```python
from build123d import *

# Parameters (mm, degrees)
OUTLINE_DEPTH        = 1.6
FILLETS_R            = 0.8
FILLET2_R            = 2
SKETCH3_R            = 8.5
LED_RING_AREA_DEPTH  = 1
SKETCH4_R            = 1.7
MOUNTING_HOLES_DEPTH = 49.37445749
SKETCH5_W            = 8.8
SKETCH5_H            = 7.25
CONNECTOR_AREA_DEPTH = 6.4


with BuildPart() as part:
    # Sketch1 → Outline (new body)
    with BuildSketch(Plane.XY):
        with BuildLine():
            Line((-16.970562748, -16.970562748), (-16.970562748, -39.970562748))
            ThreePointArc((-16.970562748, -39.970562748), (-16.384776311, -41.384776311), (-14.970562748, -41.970562748))
            Line((-14.970562748, -41.970562748), (14.970562748, -41.970562748))
            ThreePointArc((14.970562748, -41.970562748), (16.384776311, -41.384776311), (16.970562748, -39.970562748))
            Line((16.970562748, -39.970562748), (16.970562748, -16.970562748))
            ThreePointArc((16.970562748, -16.970562748), (0, 24), (-16.970562748, -16.970562748))
        make_face()
        with BuildLine():
            Line((16.377011502, 2.010844166), (12.803845356, 1.57211453))
            ThreePointArc((12.803845356, 1.57211453), (12.9, 0), (12.803845356, -1.57211453))
            Line((12.803845356, -1.57211453), (14.391919199, -1.767105479))
            ThreePointArc((14.391919199, -1.767105479), (14.084460012, -3.446445439), (13.581746744, -5.078007028))
            Line((13.581746744, -5.078007028), (15.455091123, -5.778421791))
            ThreePointArc((15.455091123, -5.778421791), (16.38562954, -1.939367058), (16.377011502, 2.010844166))
        make_face(mode=Mode.SUBTRACT)
        with BuildLine():
            Line((-16.377011502, -2.010844166), (-12.803845356, -1.57211453))
            ThreePointArc((-12.803845356, -1.57211453), (-12.9, 0), (-12.803845356, 1.57211453))
            Line((-12.803845356, 1.57211453), (-14.391919199, 1.767105479))
            ThreePointArc((-14.391919199, 1.767105479), (-14.084460012, 3.446445439), (-13.581746744, 5.078007028))
            Line((-13.581746744, 5.078007028), (-15.455091123, 5.778421791))
            ThreePointArc((-15.455091123, 5.778421791), (-16.38562954, 1.939367058), (-16.377011502, -2.010844166))
        make_face(mode=Mode.SUBTRACT)
        with BuildLine():
            ThreePointArc((-9.611831115, -11.254008291), (-7.511567772, -12.752111575), (-5.183069243, -13.862748401))
            ThreePointArc((-5.183069243, -13.862748401), (-4.713897396, -14.892252057), (-5.743401053, -15.361423904))
            ThreePointArc((-5.743401053, -15.361423904), (-8.323629153, -14.130718231), (-10.650947993, -12.470657836))
            ThreePointArc((-10.650947993, -12.470657836), (-10.739714326, -11.342774625), (-9.611831115, -11.254008291))
        make_face(mode=Mode.SUBTRACT)
        with BuildLine():
            ThreePointArc((5.743401053, 15.361423904), (4.713897396, 14.892252057), (5.183069243, 13.862748401))
            ThreePointArc((5.183069243, 13.862748401), (7.511567772, 12.752111575), (9.611831115, 11.254008291))
            ThreePointArc((9.611831115, 11.254008291), (10.739714326, 11.342774625), (10.650947993, 12.470657836))
            ThreePointArc((10.650947993, 12.470657836), (8.323629153, 14.130718231), (5.743401053, 15.361423904))
        make_face(mode=Mode.SUBTRACT)
    extrude(amount=OUTLINE_DEPTH)

    # Fillets
    fillets_edges = [part.edges().sort_by_distance(p)[0] for p in [
        (16.377011502, 2.010844166, 0.8),
        (12.803845356, 1.57211453, 0.8),
        (13.581746744, -5.078007028, 0.8),
        (15.455091123, -5.778421791, 0.8),
        (14.391919199, -1.767105479, 0.8),
        (12.803845356, -1.57211453, 0.8),
        (-12.803845356, -1.57211453, 0.8),
        (-16.377011502, -2.010844166, 0.8),
        (-15.455091123, 5.778421791, 0.8),
        (-13.581746744, 5.078007028, 0.8),
        (-12.803845356, 1.57211453, 0.8),
        (-14.391919199, 1.767105479, 0.8),
    ]]
    fillet(fillets_edges, radius=FILLETS_R - 0.0001)  # a hair under: the kernel refuses the full size

    # Fillet2
    fillet2_edges = [part.edges().sort_by_distance(p)[0] for p in [
        (16.970562748, -16.970562748, 0.8),
        (-16.970562748, -16.970562748, 0.8),
    ]]
    fillet(fillet2_edges, radius=FILLET2_R)

    # Sketch3 → LED Ring Area (add)
    with BuildSketch(Plane.XY.offset(1.6)):
        Circle(SKETCH3_R)
    extrude(amount=LED_RING_AREA_DEPTH)

    # Sketch4 → Mounting Holes (cut, through all)
    with BuildSketch(Plane.XY.offset(1.6)):
        with Locations((-11.720562748, -36.720562748)):
            Circle(SKETCH4_R)
        with Locations((11.720562748, -36.720562748)):
            Circle(SKETCH4_R)
    extrude(amount=-MOUNTING_HOLES_DEPTH, mode=Mode.SUBTRACT)

    # Sketch5 → Connector Area (add)
    with BuildSketch(Plane.XY.offset(1.6)):
        with Locations((0, -36.845562748)):
            Rectangle(SKETCH5_W, SKETCH5_H)
    extrude(amount=CONNECTOR_AREA_DEPTH)


solid = part.part
```
Geometry: final body of the model. Coordinates: model frame, mm. A direction names the side the tool comes from. Round coordinates to 2 decimals unless told otherwise and drop trailing zeros. Write each loop counter-clockwise with the first axis right and the second up, starting at its lowest first coordinate (ties: lowest second). Pieces come first, ordered by that corner, then holes. Notation, with made-up numbers: M -2,11 L 45,11 A29 cw 45,31 Z; hole C 80,23.5 d1. An arc over 180 degrees is marked long. Answer in a Markdown table with one row per item. Add a question column.
(1) Cut plane C-C, the plane x = 12. Return the cut outline in (y, z), then the cut area to 3 significant figures.
(2) Cut plane A-A, the plane y = 0. Return the cut outline in (x, z).
(3) Contact query for flat-ended pins moving along their axis: pin 1 (8.5 mm diameter, centred on x = -2.5, y = -1, fed in from +Z); pin 2 (1.9 mm diameter, centred on y = -38, z = 5, fed in from -X); pin 3 (0.5 mm diameter, centred on y = -33, z = 1, fed in from -X). Output: stop coordinate, or through.
(4) Cut plane D-D, the plane y = -22. Return the cut outline in (x, z), then the cut area to 3 significant figures.
(5) Cut plane B-B, the plane x = 0. Return the cut outline in (y, z), then the cut area to 3 significant figures.
(6) Reachability of faces 4 (the face through (0, 0, 2.6)), 5 (the face through (0, -41.971, 1)), 6 (the face through (0, -40.471, 5)), 7 (the face through (14.077, -3.477, 0.789)) from +Z, -Z, +X, -X, +Y, -Y: full face, straight path, thin tool, end or side. Return the list, or none.
(7) Ray query, L1, parallel to Y at x = 0.5, z = 2.5; L2, parallel to Z at x = -17.5, y = 10; L3, parallel to Y at x = 3, z = 6.5. Return the intervals inside material, ascending.
(8) Draft query along X for faces 1 (the face through (-7.543, -12.734, 0.789)), 2 (the face through (-16.971, -29, 1)), 3 (the face through (0, -33.221, 5)). Return one class per face: pulls with the +X half, pulls with the -X half, needs draft (parallel to the pull), parting line crosses it, or undercut.
Established:
| question | item | result |
|---|---|---|
| 1 | outline | M -41.97,0 L -38.4,0 L -38.4,1.6 L -41.97,1.6 Z; M -35.04,0 L 20.78,0 L 20.78,1.6 L -35.04,1.6 Z |
| 1 | area | 95.0 mm² |
| 2 | outline | M -24,0 L -16.5,0 L -16.5,1.6 L -24,1.6 Z; M -12.9,0 L 12.9,0 L 12.9,1.6 L 8.5,1.6 L 8.5,2.6 L -8.5,2.6 L -8.5,1.6 L -12.9,1.6 Z; M 16.5,0 L 24,0 L 24,1.6 L 16.5,1.6 Z |
| 3 | pin 1 | z = 2.6 |
| 3 | pin 2 | x = -4.4 |
| 3 | pin 3 | x = -16.97 |
| 4 | outline | M -16.97,0 L 16.97,0 L 16.97,1.6 L -16.97,1.6 Z |
| 4 | area | 54.3 mm² |
| 5 | outline | M -41.97,0 L 24,0 L 24,1.6 L 8.5,1.6 L 8.5,2.6 L -8.5,2.6 L -8.5,1.6 L -33.22,1.6 L -33.22,8 L -40.47,8 L -40.47,1.6 L -41.97,1.6 Z |
| 5 | area | 169 mm² |
| 6 | face 4 | +Z, +X, -X, +Y |
| 6 | face 5 | +Z, -Z, +X, -X, -Y |
| 6 | face 6 | +Z, +X, -X, -Y |
| 6 | face 7 | +Z, -Z |
| 7 | L1 | -40.47 to -33.22, -8.49 to 8.49 |
| 7 | L2 | 0 to 1.6 |
| 7 | L3 | -40.47 to -33.22 |
| 8 | face 1 | undercut |
| 8 | face 2 | pulls with the -X half |
| 8 | face 3 | needs draft |
